The model under review builds one solid part; all positions refer to its coordinate system, in mm. A direction names the side the tool comes from. Give positions to 0.01 mm unless a question says otherwise; leave off trailing zeros. Write each loop counter-clockwise with the first axis right and the second up, starting at its lowest first coordinate (ties: lowest second). Pieces come first, ordered by that corner, then holes. Notation, with made-up numbers: (76.25, 77) - (117.25, 77) arc R32 cw to (117.25, 109) - close; hole circle Ø1 at (52, 75.5). An arc over 180 degrees is marked (long way). Write item = value, one per line.
```python
from build123d import *

# Parameters (mm, degrees)
EXTRUDE_1_DEPTH     = 11
SKETCH_4_R          = 2.25
CUT_EXTRUDE_1_DEPTH = 10
SKETCH_2_R          = 2.25
CUT_EXTRUDE_2_DEPTH = 20
FILLET_2_R          = 0.5
RIB_2_REACH         = 36.249
SKETCH_5_WALL_W     = 84.92038026
SKETCH_5_WALL_H     = 3
RIB_3_REACH         = 36.249
SKETCH_6_WALL_W     = 84.92038026
SKETCH_6_WALL_H     = 3
FILLET_3_R          = 3


with BuildPart() as part:
    # 草图1 → 凸台-拉伸1 (new, symmetric)
    with BuildSketch(Plane.XY):
        with BuildLine():
            Line((-17, 0), (-17, -15))
            ThreePointArc((-17, -15), (-17.585786438, -16.414213562), (-19, -17))
            Line((-19, -17), (-19.5, -17))
            ThreePointArc((-19.5, -17), (-19.853553391, -16.853553391), (-20, -16.5))
            Line((-20, -16.5), (-20, 3))
            Line((-20, 3), (-0.5, 3))
            ThreePointArc((-0.5, 3), (-0.146446609, 2.853553391), (0, 2.5))
            Line((0, 2.5), (0, 2))
            ThreePointArc((0, 2), (-0.585786438, 0.585786438), (-2, 0))
            Line((-2, 0), (-17, 0))
        make_face()
    extrude(amount=EXTRUDE_1_DEPTH, both=True)

    # 草图4 → 切除-拉伸1 (cut)
    with BuildSketch(Plane(origin=(0, 0, 0), x_dir=(1, 0, 0), z_dir=(0, 1, 0))):
        with Locations((-5, -2.5)):
            Circle(SKETCH_4_R)
        with Locations((-12, 2.5)):
            Circle(SKETCH_4_R)
    extrude(amount=CUT_EXTRUDE_1_DEPTH, mode=Mode.SUBTRACT)

    # 草图2 → 切除-拉伸2 (cut)
    with BuildSketch(Plane(origin=(-17, 0, 0), x_dir=(0, 0, -1), z_dir=(1, 0, 0))):
        with Locations((2.5, -12)):
            Circle(SKETCH_2_R)
        with Locations((-2.5, -5)):
            Circle(SKETCH_2_R)
    extrude(amount=-CUT_EXTRUDE_2_DEPTH, mode=Mode.SUBTRACT)

    # 圆角2
    fillet_2_edges = [part.edges().sort_by_distance(p)[0] for p in [
        (-7.25, 0, 2.5),
        (-14.25, 0, -2.5),
        (-17, -12, -0.25),
        (-17, -5, 4.75),
    ]]
    fillet(fillet_2_edges, radius=FILLET_2_R)

    # 草图5 wall → 筋2 (add, up to next)
    with BuildSketch(Plane(origin=(-13, -6, -11), x_dir=(-0.554700196225, -0.832050294338, 0), z_dir=(0.832050294338, -0.554700196225, 0)), mode=Mode.PRIVATE) as rib_2_sk1:
        with Locations((0, -1.5)):
            Rectangle(SKETCH_5_WALL_W, SKETCH_5_WALL_H)
    rib_2_tool1 = extrude(rib_2_sk1.sketch, amount=-RIB_2_REACH, mode=Mode.PRIVATE) - part.part
    add(rib_2_tool1.solids().sort_by_distance((-13, -6, -11))[0])

    # 草图6 wall → 筋3 (add, up to next)
    with BuildSketch(Plane(origin=(-13, -6, 11), x_dir=(-0.554700196225, -0.832050294338, 0), z_dir=(-0.832050294338, 0.554700196225, 0)), mode=Mode.PRIVATE) as rib_3_sk1:
        with Locations((0, -1.5)):
            Rectangle(SKETCH_6_WALL_W, SKETCH_6_WALL_H)
    rib_3_tool1 = extrude(rib_3_sk1.sketch, amount=RIB_3_REACH, mode=Mode.PRIVATE) - part.part
    add(rib_3_tool1.solids().sort_by_distance((-13, -6, 11))[0])

    # 圆角3
    fillet_3_edges = [part.edges().sort_by_distance(p)[0] for p in [
        (-20, 3, 0),
        (-17, -12, -9.5),
        (-9, 0, -9.5),
        (-17, -12, 9.5),
        (-9, 0, 9.5),
    ]]
    fillet(fillet_3_edges, radius=FILLET_3_R)


solid = part.part
```
1. For line 1 (Z direction, x = -10.75, y = -2.25); line 2 (Z direction, x = -5, y = 1.05); line 3 (X direction, y = -2, z = 7), list the stretches that pass through material, from the lowest coordinate up. Write a range as from..to.
Findings below:
line_1 = -11..-8, 8..11
line_2 = -11..0.25, 4.75..11
line_3 = -20..-17
2. Take a section at D-D on z = 7.5. Give the boundary of the cut face in (x, y), and give its area (3 significant figures).
Findings below:
outline = (-20, -16.5) arc R0.5 ccw to (-19.5, -17) - (-19, -17) arc R2 ccw to (-17, -15) - (-17, 0) - (-2, 0) arc R2 ccw to (0, 2) - (0, 2.5) arc R0.5 ccw to (-0.5, 3) - (-17, 3) arc R3 ccw to (-20, 0) - close
area = 107 mm²
3. Take a section at A-A on x = -5. Give the boundary of the cut face in (y, z), and give its area (3 significant figures).
Findings below:
outline = (0, -11) - (3, -11) - (3, 0.25) - (0.5, 0.25) arc R0.5 ccw to (0, -0.25) - close; (0, 5.25) arc R0.5 ccw to (0.5, 4.75) - (3, 4.75) - (3, 11) - (0, 11) - close
area = 52.4 mm²
4. Machinability: for faces 1 (the flat face through (-15, -4, 8)), 2 (the cylindrical face through (-2.92, 1.73, 3.36)), which of the approach directions +Z, -Z, +X, -X, +Y, -Y give a long, thin tool a straight path to every point of the face, cutting with its end or side? Answer none if there is none.
Findings below:
face_1 = +X, -Y
face_2 = +Y, -Y
5. Take a section at C-C on y = -12. Give the boundary of the cut face in (x, z).
Findings below:
outline = (-20, -11) - (-16.86, -11) - (-16.86, -8) - (-17, -8) - (-17, -5.25) arc R0.5 ccw to (-17.5, -4.75) - (-20, -4.75) - close; (-20, -0.25) - (-17.5, -0.25) arc R0.5 ccw to (-17, 0.25) - (-17, 8) - (-16.86, 8) - (-16.86, 11) - (-20, 11) - close
6. Take a section at B-B on z = 2.5. Give the boundary of the cut face in (x, y).
Findings below:
outline = (-20, -16.5) arc R0.5 ccw to (-19.5, -17) - (-19, -17) arc R2 ccw to (-17, -15) - (-17, -7.75) arc R0.5 ccw to (-17.5, -7.25) - (-20, -7.25) - close; (-20, -2.75) - (-17.5, -2.75) arc R0.5 ccw to (-17, -2.25) - (-17, 0) - (-7.75, 0) arc R0.5 ccw to (-7.25, 0.5) - (-7.25, 3) - (-17, 3) arc R3 ccw to (-20, 0) - close; (-2.75, 0.5) arc R0.5 ccw to (-2.25, 0) - (-2, 0) arc R2 ccw to (0, 2) - (0, 2.5) arc R0.5 ccw to (-0.5, 3) - (-2.75, 3) - close
7. Draft analysis for pull direction Z (two halves, no side actions). For faces 3 (the flat face through (-17, -7, 0)), 4 (the flat face through (-20, -8, 0)), 5 (the flat face through (-14, -3, 11)), 6 (the flat face through (-15, -4, -8)), state which applies: +Z half, -Z half, draft (parallel to the pull), parting line (faces both ways), or undercut.
Findings below:
face_3 = undercut
face_4 = draft
face_5 = +Z half
face_6 = undercut
8. Insertion check: P1, Ø4, axis at y = -6, z = -6.5, coming from the +X side; P2, Ø2.5, axis at x = -5, z = 2.5, coming from the +Y side; P3, Ø7.5, axis at x = -8.5, z = -4, coming from the -Y side; P4, Ø1, axis at x = -17.5, z = -3.5, coming from the -Y side. Each pin has a flat end and moves straight along its axis. Give the tip position at first contact, or say it passes through.
Findings below:
P1 = -12.12
P2 = through
P3 = 0
P4 = -16.73
